Could you check a few things on this drawing? It's one solid part, dimensions in mm from its lowest x, y, z. A direction names the side the tool comes from. Coordinates: 2 decimals unless noted, no trailing zeros. Loops run counter-clockwise (first coordinate to the right, second up) from the corner with the lowest first, then second, coordinate; pieces in that order, holes last.
1) Will these pins go through, and if not, where does the flat tip stop? P1, Ø12, axis at y = 19.5, z = 4.5, coming from the +X side; P2, Ø12, axis at y = 4.5, z = 3.5, coming from the -X side; P3, Ø5, axis at y = 3.5, z = 15.5, coming from the +X side; P4, Ø5, axis at x = 34.5, y = 23, coming from the +Z side.
2) Imagine slicing it at A-A on y = 3. Please give me the cut outline in (x, z).
3) Thinking about a two-plate mould opening in X: for the marked faces 4, 5, 6 and 7, which applies, released by +X, released by -X, zero draft, split by the parting line, or undercut?
4) If I drill on line 1 along Z through (x, y) = (8, 27.5); line 2 along Y through (x, z) = (27, 17.5); line 3 along X through (y, z) = (28, 8.5), over which ranges is the centre line in solid material (lowest first)?
5) Imagine slicing it at C-C on y = 26.25. Please give me the cut outline in (x, z).
6) Imagine slicing it at D-D on z = 17.25. Please give me the cut outline in (x, y), plus the area to 3 significant figures.
7) Imagine slicing it at B-B on x = 8. Please give me the cut outline in (y, z).
8) For the marked faces 1, 2 and 3, which set-ups out of +Z, -Z, +X, -X, +Y, -Y let a thin tool reach every point of the face, with its end or its side?
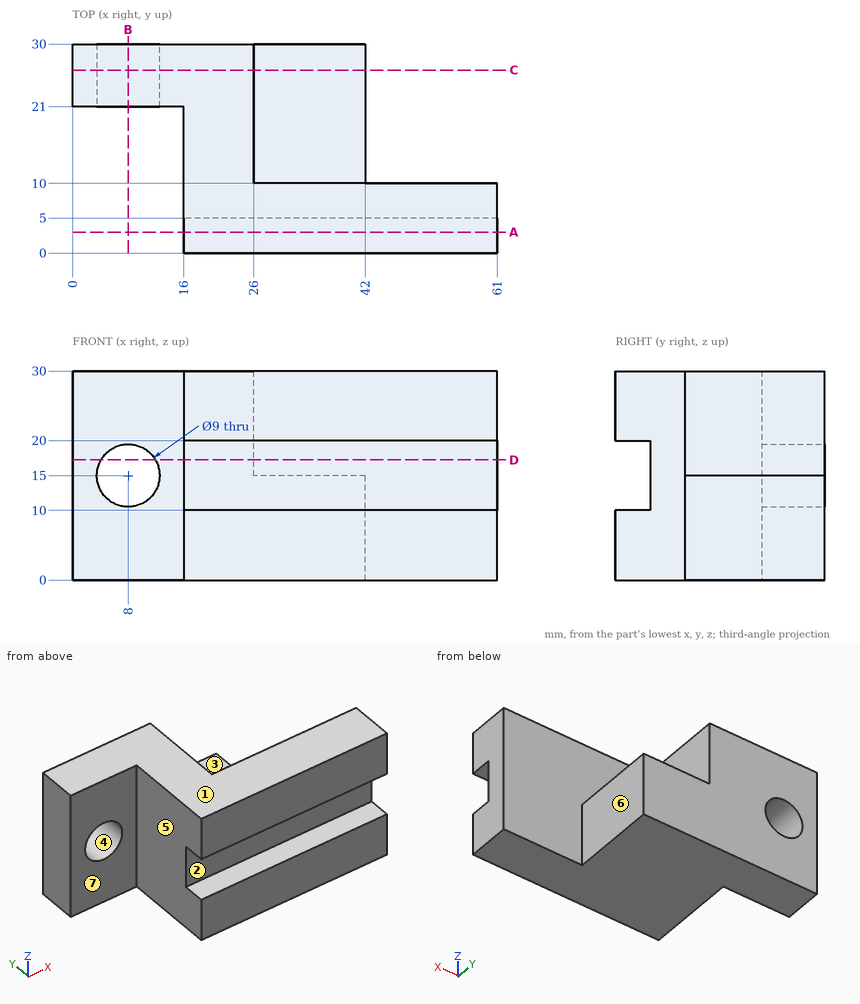
Filled in:
1. P1: stops at x = 42
1. P2: stops at x = 16
1. P3: stops at x = 61
1. P4: stops at z = 15
2. outline: (16, 0) - (61, 0) - (61, 10) - (16, 10) - close; (16, 20) - (61, 20) - (61, 30) - (16, 30) - close
3. face 4: undercut
3. face 5: released by -X
3. face 6: released by +X
3. face 7: zero draft
4. line 1: z = 0 to 10.5, 19.5 to 30
4. line 2: y = 5 to 10
4. line 3: x = 0 to 42
5. outline: (0, 0) - (42, 0) - (42, 15) - (26, 15) - (26, 30) - (0, 30) - close; hole circle Ø9 at (8, 15)
6. outline: (0, 21) - (4.1, 21) - (4.1, 30) - (0, 30) - close; (11.9, 21) - (16, 21) - (16, 5) - (61, 5) - (61, 10) - (26, 10) - (26, 30) - (11.9, 30) - close
6. area: 499 mm2
7. outline: (21, 0) - (30, 0) - (30, 10.5) - (21, 10.5) - close; (21, 19.5) - (30, 19.5) - (30, 30) - (21, 30) - close
8. face 1: +Z, +X, -X, +Y, -Y
8. face 2: +X, -X, -Y
8. face 3: +Z, +X, +Y
